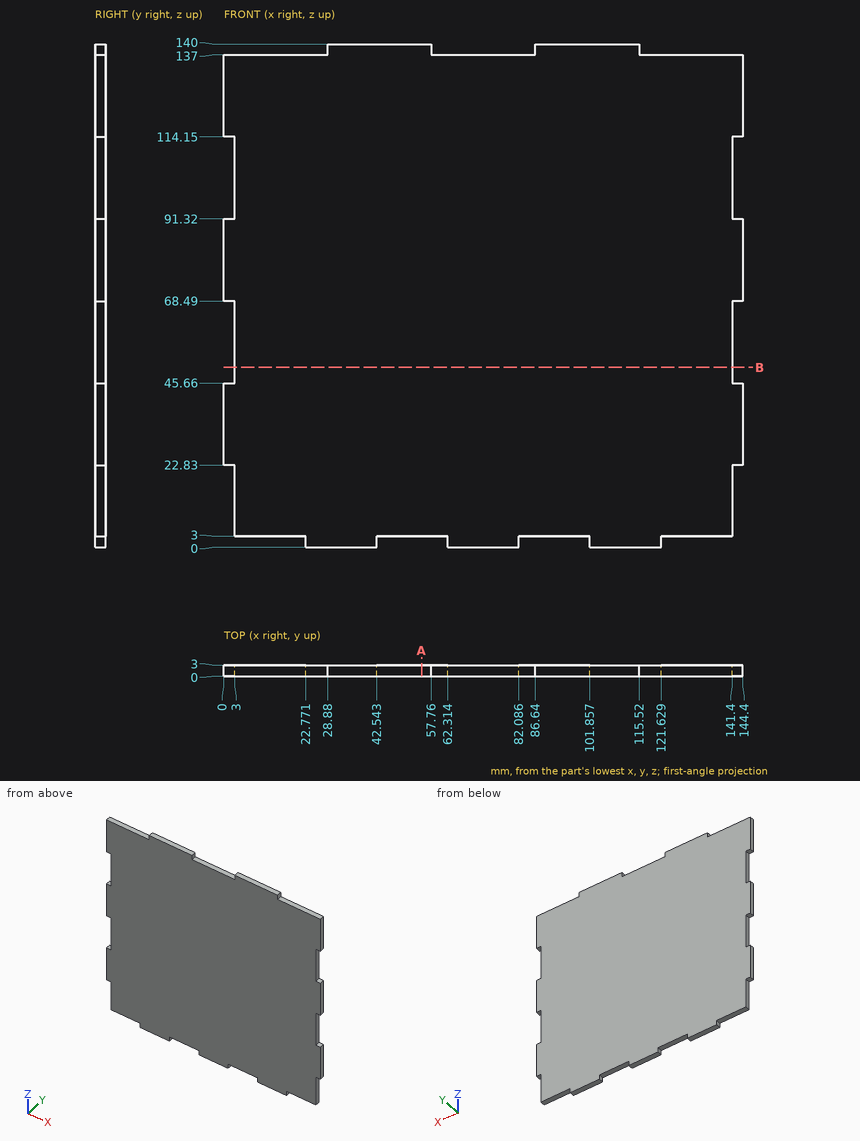
Source: three-view drawing plus pictorial views. Frame: mm from the lowest corner of the part. Round coordinates to 2 decimals unless told otherwise and drop trailing zeros. Loops run counter-clockwise (first coordinate to the right, second up) from the corner with the lowest first, then second, coordinate; pieces in that order, holes last. Notation, with made-up numbers: M -14.5,-19 L 14.5,-19 A21 cw 14.5,-12 Z; hole C -38.5,75.5 d9. An arc over 180 degrees is marked long. Answer as CSV lines item,"result". Start each with the question number.
(1) First-contact query: pin 1 (1.5 mm diameter, centred on y = 1.5, z = 138.5, fed in from +X); pin 2 (0.9 mm diameter, centred on y = 2, z = 17, fed in from -X); pin 3 (1.5 mm diameter, centred on x = 120, z = 62, fed in from -Y); pin 4 (1.5 mm diameter, centred on x = 142.5, y = 1, fed in from -Z). Flat tips, straight axial feed; report the tip coordinate or a pass-through.
(2) Line query: line 1 (Z direction, x = 121.5, y = 2.6); line 2 (X direction, y = 2.65, z = 14); line 3 (Z direction, x = 15, y = 1.5). Output: solid intervals per line, ascending. Write a range as [from, to].
(3) Section A-A, the plane x = 55. Output: boundary loops of the cut face in (y, z).
(4) Section B-B, the plane z = 50. Output: boundary loops of the cut face in (x, y).
Values found:
1,pin 1,"stops at x = 115.52"
1,pin 2,"stops at x = 3"
1,pin 3,"stops at y = 0"
1,pin 4,"stops at z = 22.83"
2,line 1,"z = [0, 137]"
2,line 2,"x = [3, 141.4]"
2,line 3,"z = [3, 137]"
3,outline,"M 0,3 L 3,3 L 3,140 L 0,140 Z"
4,outline,"M 3,0 L 141.4,0 L 141.4,3 L 3,3 Z"
